Autodesk Inventor part; units mm, degrees
ref_plane "YZ Plane" through (0, 0, 0) normal (1, 0, 0) x (0, 1, 0)
ref_plane "XZ Plane" through (0, 0, 0) normal (0, 1, 0) x (-1, 0, 0)
ref_plane "XY Plane" through (0, 0, 0) normal (0, 0, 1) x (1, 0, 0)
sketch "Sketch1" plane through (0, 0, 0) normal (0, 0, 1) x (1, 0, 0)
  line L0 (-10.627, -30.5907) -> (-13.477, -30.5907)
  line L1 (-10.627, -30.5907) -> (-10.627, -40.5907)
  line L2 (-10.627, -40.5907) -> (-12.127, -40.5907)
  line L3 (-12.127, -40.5907) -> (-12.127, -30.5907)
  line L4 (-10.627, -30.5907) -> (-10.627, -26.5988)
  line L5 (-13.477, -30.5907) -> (-13.477, -30.2107)
  line L6 (-13.477, -30.2107) -> (-13.477, -28.9407)
  line L7 (-13.477, -28.9407) -> (-10.627, -28.9407)
  point P0 (0, 0)
  dimension "d0" = 2.85
  dimension "d2" = 10
  dimension "d3" = 1.5
  dimension "d18" = 0.38
  dimension "d19" = 1.65
revolve "Revolution1" add sketch "Sketch1" angle 360 about axis through (-10.627, -30.5907, 0) along (0, -1, 0)
chamfer "Chamfer2" distance 0.2 angle 45 1 edges at (-9.127, -40.5907, 0)
fillet "Empalme2" radius 1.27 1 edges at (-7.777, -28.9407, 0)
sketch "Boceto2" plane through (-10.627, -28.9407, 0) normal (0, 1, 0) x (1, 0, 0)
  line L0 (0.8985, 0.7252) -> (1.0773, -0.4156)
  line L1 (1.0773, -0.4156) -> (0.1788, -1.1408)
  line L2 (0.1788, -1.1408) -> (-0.8985, -0.7252)
  line L3 (-0.8985, -0.7252) -> (-1.0773, 0.4156)
  line L4 (-1.0773, 0.4156) -> (-0.1788, 1.1408)
  line L5 (-0.1788, 1.1408) -> (0.8985, 0.7252)
  point P0 (10.627, 0)
  point P1 (0, 0)
  dimension "d21" = 2
extrude "Extrusión1" cut sketch "Boceto2" against normal blind 1.3
thread "Rosca2"
properties part number "Tornillo Allen cabeeza botón M3x10mm"
Geometry check sheet. Reference: the model listing, model coordinates, mm. A direction names the side the tool comes from. Give positions to 0.01 mm unless a question says otherwise; leave off trailing zeros. Order: outer loops, then holes, each group sorted by start corner. A loop starts at its lowest first (then second) coordinate and runs counter-clockwise, first axis right, second up.
1. Release check for a two-part mould opening along X. For faces 1 (the face through (-11, -40.591, 0)), 2 (the face through (-12, -35.4, -0.6)), 3 (the face through (-11, -30.241, 0)) record: pulls with the +X half, pulls with the -X half, needs draft (parallel to the pull), parting line crosses it, or undercut.
2. Section check B-B, the plane z = 0. Enter the section's corners in (x, y), and give its area (3 significant figures).
3. Section check A-A, the plane y = -30. Enter the section's corners in (x, z).
4. Gauge pin test, flat ends, axial feed: pin 1 Ø1.1 at (x, z) = (-10.5, 0) entering from +Y; pin 2 Ø2 at (y, z) = (-37, 1) entering from +X; pin 3 Ø3 at (x, y) = (-11.5, -34) entering from -Z. Record the tip position at first contact, or that the pin passes through.
5. Thickness scan on L1, parallel to Z at x = -10.1, y = -29.75; L2, parallel to X at y = -29.75, z = 0.6; L3, parallel to Z at x = -11, y = -36.25. Record the ranges inside material, lowest first.
6. Access from +Z, -Z, +X, -X, +Y, -Y to the whole of each face (thin tool, end or side, straight path). Record for faces 4 (the face through (-12, -28.941, 0)), 5 (the face through (-9.99, -29.58, 0.77)), 6 (the face through (-12, -30.591, 1)).
7. Section check C-C, the plane y = -35. Enter the section's corners in (x, z), and give its area (3 significant figures).
Values follow:
1. face 1: needs draft
1. face 2: parting line crosses it
1. face 3: undercut
2. outline: (-13.48, -30.59) - (-12.13, -30.59) - (-12.13, -40.39) - (-11.93, -40.59) - (-9.33, -40.59) - (-9.13, -40.39) - (-9.13, -30.59) - (-7.78, -30.59) - (-7.78, -30.21) arc R1.27 ccw to (-9.05, -28.94) - (-9.61, -28.94) - (-9.61, -30.24) - (-11.64, -30.24) - (-11.64, -28.94) - (-12.21, -28.94) arc R1.27 ccw to (-13.48, -30.21) - close
2. area: 36.0 mm2
3. outline: circle Ø5.66 at (-10.63, 0); hole (-11.7, -0.42) - (-10.81, -1.14) - (-9.73, -0.73) - (-9.55, 0.42) - (-10.45, 1.14) - (-11.53, 0.73) - close
4. pin 1: stops at y = -30.24
4. pin 2: stops at x = -9.13
4. pin 3: stops at z = -1.5
5. L1: z = -2.71 to -0.87, 0.86 to 2.71
5. L2: x = -13.32 to -11.55, -9.78 to -7.93
5. L3: z = -1.45 to 1.45
6. face 4: +Z, -Z, +X, -X, +Y
6. face 5: +Y
6. face 6: -Y
7. outline: circle Ø3 at (-10.63, 0)
7. area: 7.07 mm2
